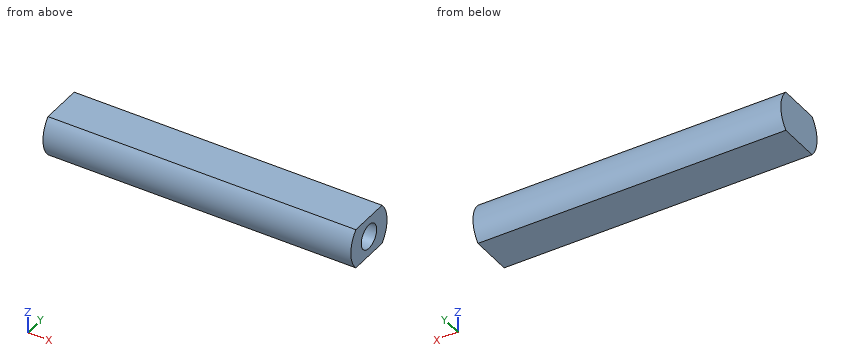
from build123d import *

# Parameters (mm, degrees)
F0_R     = 4.7625
F1_DEPTH = 50.8
F3_DEPTH = 50.801
F4_R     = 2.0193
F5_DEPTH = 44.45


# Not quite as in the source:
# - a pattern or mirror of a feature is missing from the dataset's text; its kind, count and spacing are read off the source's solid


with BuildPart() as f1:
    # F0 (on Right) → F1 (new body)
    with BuildSketch(Plane.YZ):
        Circle(F0_R)
    extrude(amount=F1_DEPTH)

    # F2 (on face) → F3 (cut, through all)
    with BuildSketch(Plane.YZ.offset(50.8)):
        with BuildLine():
            Line((-3.444112623, 3.2893), (3.444112623, 3.2893))
            ThreePointArc((3.444112623, 3.2893), (0, 4.7625), (-3.444112623, 3.2893))
        make_face()
    f3 = extrude(amount=-F3_DEPTH, mode=Mode.SUBTRACT)

    # F3_copies: F3 across plane
    add(f3.mirror(Plane(origin=(0, 0, 0), x_dir=(-1, 0, 0), z_dir=(0, 0, -1))), mode=Mode.SUBTRACT)

    # F4 (on face) → F5 (cut)
    with BuildSketch(Plane.YZ.offset(50.8)):
        Circle(F4_R)
    extrude(amount=-F5_DEPTH, mode=Mode.SUBTRACT)


solid = f1.part
Geometry check sheet. Reference: the model listing, model coordinates, mm. Coordinates: 2 decimals unless noted, no trailing zeros. Order: outer loops, then holes, each group sorted by start corner. A loop starts at its lowest first (then second) coordinate and runs counter-clockwise, first axis right, second up. Notation, with made-up numbers: (-23, 37) -> (-4, 37) arc R28 ccw to (-4, 71) -> close; hole circle Ø8 at (2.25, 3). An arc over 180 degrees is marked (long way). Use a Markdown table: item, result. Add a question column.
1. Go/stop test with a flat-tipped pin: pin 1 Ø1 at (x, z) = (30, -1.5) entering from -Y. Record where the tip stops, or that it passes through.
2. Cross-section at B-B (z = 0). Enter the section's corners in (x, y), and give its area (3 significant figures).
3. Cross-section at C-C (y = 0). Enter the section's corners in (x, z), and give its area (3 significant figures).
4. Material ranges on L1, parallel to Z at x = 33, y = 0; L2, parallel to Y at x = 14.5, z = -0.75; L3, parallel to X at y = -0.5, z = -1.25, recorded low to high.
5. Cross-section at A-A (x = 28). Enter the section's corners in (y, z) (1 decimal), and give its area (3 significant figures).
Filled sheet:
| question | item | result |
|---|---|---|
| 1 | pin 1 | y = -4.66 |
| 2 | outline | (0, -4.76) -> (50.8, -4.76) -> (50.8, -2.02) -> (6.35, -2.02) -> (6.35, 2.02) -> (50.8, 2.02) -> (50.8, 4.76) -> (0, 4.76) -> close |
| 2 | area | 304 mm2 |
| 3 | outline | (0, -3.29) -> (50.8, -3.29) -> (50.8, -2.02) -> (6.35, -2.02) -> (6.35, 2.02) -> (50.8, 2.02) -> (50.8, 3.29) -> (0, 3.29) -> close |
| 3 | area | 155 mm2 |
| 4 | L1 | -3.29 to -2.02, 2.02 to 3.29 |
| 4 | L2 | -4.7 to -1.87, 1.87 to 4.7 |
| 4 | L3 | 0 to 6.35 |
| 5 | outline | (-3.4, -3.3) -> (3.4, -3.3) arc R4.8 ccw to (3.4, 3.3) -> (-3.4, 3.3) arc R4.8 ccw to start; hole circle Ø4 at (0, 0) |
| 5 | area | 44.4 mm2 |
